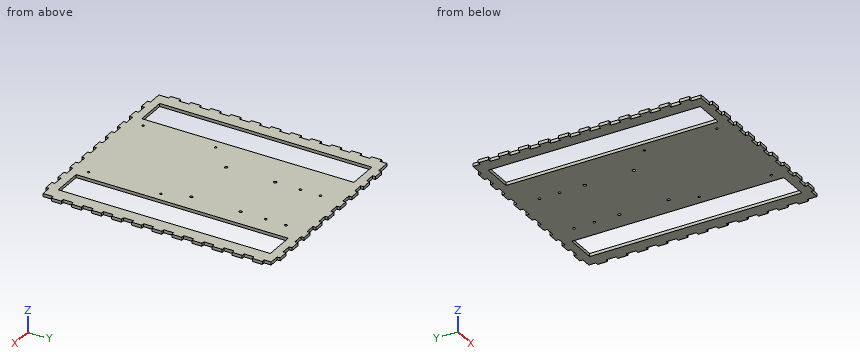
from build123d import *

# Parameters (mm, degrees)
SKETCH1_W           = 194
SKETCH1_H           = 227
BOSS_EXTRUDE1_DEPTH = 3
SKETCH2_W           = 3
SKETCH2_H           = 10
BOSS_EXTRUDE2_DEPTH = 3
LPATTERN1_COUNT     = 11
LPATTERN1_PITCH     = 20
SKETCH4_W           = 3
SKETCH4_H           = 10
BOSS_EXTRUDE3_DEPTH = 3
LPATTERN2_COUNT     = 11
LPATTERN2_PITCH     = 20
SKETCH5_W           = 10
SKETCH5_H           = 3
BOSS_EXTRUDE4_DEPTH = 3
LPATTERN3_COUNT     = 9
LPATTERN3_PITCH     = 20
SKETCH6_W           = 10
SKETCH6_H           = 3
BOSS_EXTRUDE5_DEPTH = 3
LPATTERN4_COUNT     = 9
LPATTERN4_PITCH     = 20
SKETCH7_W           = 30
SKETCH7_H           = 211
CUT_EXTRUDE1_DEPTH  = 4
SKETCH8_R           = 1.1
SKETCH8_R_2         = 1.5
SKETCH8_R_3         = 1.25
SKETCH8_W           = 30
SKETCH8_H           = 211
CUT_EXTRUDE2_DEPTH  = 4


with BuildPart() as part:
    # Sketch1 → Boss-Extrude1 (new body)
    with BuildSketch(Plane.XY):
        with Locations((97, 113.5)):
            Rectangle(SKETCH1_W, SKETCH1_H)
    extrude(amount=BOSS_EXTRUDE1_DEPTH)

    # Sketch2 → Boss-Extrude2 (add)
    with BuildSketch(Plane(origin=(194, 0, 0), x_dir=(0, 0, -1), z_dir=(1, 0, 0))):
        with Locations((-1.5, 15)):
            Rectangle(SKETCH2_W, SKETCH2_H)
    boss_extrude2 = extrude(amount=BOSS_EXTRUDE2_DEPTH)

    # LPattern1: Boss-Extrude2 ×11
    with Locations(*[(0, i * LPATTERN1_PITCH, 0) for i in range(1, LPATTERN1_COUNT)]):
        add(boss_extrude2)

    # Sketch4 → Boss-Extrude3 (add)
    with BuildSketch(Plane.ZY):
        with Locations((1.5, 15)):
            Rectangle(SKETCH4_W, SKETCH4_H)
    boss_extrude3 = extrude(amount=BOSS_EXTRUDE3_DEPTH)

    # LPattern2: Boss-Extrude3 ×11
    with Locations(*[(0, i * LPATTERN2_PITCH, 0) for i in range(1, LPATTERN2_COUNT)]):
        add(boss_extrude3)

    # Sketch5 → Boss-Extrude4 (add)
    with BuildSketch(Plane.XZ):
        with Locations((179, 1.5)):
            Rectangle(SKETCH5_W, SKETCH5_H)
    boss_extrude4 = extrude(amount=BOSS_EXTRUDE4_DEPTH)

    # LPattern3: Boss-Extrude4 ×9
    with Locations(*[(-i * LPATTERN3_PITCH, 0, 0) for i in range(1, LPATTERN3_COUNT)]):
        add(boss_extrude4)

    # Sketch6 → Boss-Extrude5 (add)
    with BuildSketch(Plane(origin=(0, 227, 0), x_dir=(1, 0, 0), z_dir=(0, 1, 0))):
        with Locations((179, -1.5)):
            Rectangle(SKETCH6_W, SKETCH6_H)
    boss_extrude5 = extrude(amount=BOSS_EXTRUDE5_DEPTH)

    # LPattern4: Boss-Extrude5 ×9
    with Locations(*[(-i * LPATTERN4_PITCH, 0, 0) for i in range(1, LPATTERN4_COUNT)]):
        add(boss_extrude5)

    # Sketch7 → Cut-Extrude1 (cut, through all)
    with BuildSketch(Plane.XY.offset(3)):
        with Locations((27, 113.5)):
            Rectangle(SKETCH7_W, SKETCH7_H)
    extrude(amount=-CUT_EXTRUDE1_DEPTH, mode=Mode.SUBTRACT)

    # Sketch8 → Cut-Extrude2 (cut, through all)
    with BuildSketch(Plane.XY.offset(3)):
        with Locations((143, 15)):
            Circle(SKETCH8_R)
        with Locations((51.5, 15)):
            Circle(SKETCH8_R)
        with Locations((143, 87)):
            Circle(SKETCH8_R)
        with Locations((51.5, 87)):
            Circle(SKETCH8_R)
        with Locations((134, 112)):
            Circle(SKETCH8_R_2)
        with Locations((76, 112)):
            Circle(SKETCH8_R_2)
        with Locations((134, 161)):
            Circle(SKETCH8_R_2)
        with Locations((76, 161)):
            Circle(SKETCH8_R_2)
        with Locations((76, 186)):
            Circle(SKETCH8_R_3)
        with Locations((76, 206)):
            Circle(SKETCH8_R_3)
        with Locations((134, 186)):
            Circle(SKETCH8_R_3)
        with Locations((134, 206)):
            Circle(SKETCH8_R_3)
        with Locations((167, 113.5)):
            Rectangle(SKETCH8_W, SKETCH8_H)
    extrude(amount=-CUT_EXTRUDE2_DEPTH, mode=Mode.SUBTRACT)


solid = part.part
The model under review builds one solid part; all positions refer to its coordinate system, in mm. Round coordinates to 2 decimals unless told otherwise and drop trailing zeros. Loops run counter-clockwise (first coordinate to the right, second up) from the corner with the lowest first, then second, coordinate; pieces in that order, holes last. Notation, with made-up numbers: (70, 64.25) - (96, 64.25) arc R16 ccw to (96, 91.25) - close; hole circle Ø5 at (17, -25). An arc over 180 degrees is marked (long way). Use CSV: the item, a comma, the result in double quotes.
(1) Take a section at A-A, the plane y = 33.5. Give the boundary of the cut face in (x, z), plus the area to 3 significant figures.
Working result:
outline,"(-3, 0) - (12, 0) - (12, 3) - (-3, 3) - close; (42, 0) - (152, 0) - (152, 3) - (42, 3) - close; (182, 0) - (197, 0) - (197, 3) - (182, 3) - close"
area,"420 mm^2"
(2) Clearance check with flat-ended pins moving along their axes: P1, Ø0.9, axis at y = 228, z = 1, coming from the -X side; P2, Ø1.5, axis at x = -2, z = 2, coming from the +Y side; P3, Ø1.5, axis at x = 70, z = 1.5, coming from the -Y side. State where each tip first meets the part, or that it passes through.
Working result:
P1,"stops at x = 14"
P2,"stops at y = 220"
P3,"stops at y = 0"
(3) For line 1 (Y direction, x = 76, z = 0.7); line 2 (X direction, y = 108, z = 2.8); line 3 (X direction, y = 34.5, z = 2.6), list the stretches that pass through material, from the lowest coordinate up.
Working result:
line 1,"y = -3 to 110.5, 113.5 to 159.5, 162.5 to 184.75, 187.25 to 204.75, 207.25 to 230"
line 2,"x = 0 to 12, 42 to 152, 182 to 194"
line 3,"x = -3 to 12, 42 to 152, 182 to 197"
(4) Take a section at C-C, the plane z = 1.75. State how many separate pieces and enclosed holes the cut face has, plus the area to 3 significant figures.
Working result:
separate pieces,"1"
enclosed holes,"14"
area,"32,500 mm^2"
(5) Take a section at B-B, the plane y = 143. Give the boundary of the cut face in (x, z).
Working result:
outline,"(0, 0) - (12, 0) - (12, 3) - (0, 3) - close; (42, 0) - (152, 0) - (152, 3) - (42, 3) - close; (182, 0) - (194, 0) - (194, 3) - (182, 3) - close"
(6) Take a section at D-D, the plane x = 91.5. Give the boundary of the cut face in (y, z).
Working result:
outline,"(0, 0) - (227, 0) - (227, 3) - (0, 3) - close"
